Part model, mm, in its own coordinate system. A direction names the side the tool comes from. Coordinates: 2 decimals unless noted, no trailing zeros. Loops run counter-clockwise (first coordinate to the right, second up) from the corner with the lowest first, then second, coordinate; pieces in that order, holes last.
```python
from build123d import *

# Parameters (mm, degrees)
REVOLVE1_ANGLE      = 180
CUT_EXTRUDE1_DEPTH  = 173.874496063
BOSS_EXTRUDE1_DEPTH = 100
CUT_EXTRUDE2_DEPTH  = 161.866404199
CUT_REVOLVE2_ANGLE  = 90
SKETCH7_R           = 25
CUT_EXTRUDE3_DEPTH  = 161.866404199
SHELL1_T            = -2


with BuildPart() as part:
    # Sketch1 → Revolve1 (revolve)
    with BuildSketch(Plane(origin=(0, 0, 0), x_dir=(0, 0, -1), z_dir=(1, 0, 0))):
        with BuildLine():
            Line((0, -55), (0, 55))
            Line((0, 55), (-76.60153846, 55))
            ThreePointArc((-76.60153846, 55), (-94.301620847, 0), (-76.60153846, -55))
            Line((-76.60153846, -55), (0, -55))
        make_face()
    revolve(axis=Axis((0, -55, 0), (0, 1, 0)), revolution_arc=REVOLVE1_ANGLE)

    # Sketch2 → Cut-Extrude1 (cut, through all)
    with BuildSketch(Plane.XZ.offset(55)):
        Polygon((0, 0), (17.67766953, 17.67766953), (110.975280637, -75.619941577), (110.975280637, 155.951540754), (-110.127783366, 155.951540754), (-110.127783366, 0), align=None)
    extrude(amount=-CUT_EXTRUDE1_DEPTH, mode=Mode.SUBTRACT)

    # Sketch3 → Boss-Extrude1 (add)
    with BuildSketch(Plane(origin=(100, 0, 0), x_dir=(0, 0, -1), z_dir=(1, 0, 0))):
        Polygon((-71.226029464, -15), (-71.226029464, 15), (39.011689542, 30), (39.011689542, -30), align=None)
    extrude(amount=-BOSS_EXTRUDE1_DEPTH)

    # Sketch4 → Cut-Revolve1 (revolve, cut)
    with BuildSketch(Plane(origin=(0, 0, 0), x_dir=(0, 0, -1), z_dir=(1, 0, 0))):
        with BuildLine():
            Line((-59.361204271, 58.010752688), (-134.505556561, 58.010752688))
            ThreePointArc((-134.505556561, 58.010752688), (-146.4820541, 0), (-134.505556561, -58.010752688))
            Line((-134.505556561, -58.010752688), (-59.361204271, -58.010752688))
            ThreePointArc((-59.361204271, -58.010752688), (-83, 0), (-59.361204271, 58.010752688))
        make_face()
    revolve(axis=Axis((0, 0, 0), (0, 1, 0)), mode=Mode.SUBTRACT)

    # Sketch5 → Cut-Extrude2 (cut, through all)
    with BuildSketch(Plane.XZ.offset(55)):
        Polygon((0, 0), (70.470143291, 80), (-50.338034401, 80), (-50.338034401, 0), align=None)
    extrude(amount=-CUT_EXTRUDE2_DEPTH, mode=Mode.SUBTRACT)

    # Sketch6 → Cut-Revolve2 (revolve, cut)
    with BuildSketch(Plane(origin=(0, 0, 0), x_dir=(0, 0, -1), z_dir=(1, 0, 0))):
        with BuildLine():
            Line((-48.985500868, 65.760327742), (-101.43758046, 65.760327742))
            ThreePointArc((-101.43758046, 65.760327742), (-120.888392471, 0), (-101.43758046, -65.760327742))
            Line((-101.43758046, -65.760327742), (-48.985500868, -65.760327742))
            ThreePointArc((-48.985500868, -65.760327742), (-82, 0), (-48.985500868, 65.760327742))
        make_face()
    revolve(axis=Axis((0, 0, 0), (0, 1, 0)), revolution_arc=CUT_REVOLVE2_ANGLE, mode=Mode.SUBTRACT)

    # Sketch7 → Cut-Extrude3 (cut, through all)
    with BuildSketch(Plane.XZ.offset(55)):
        with Locations((0, -28)):
            Circle(SKETCH7_R)
    extrude(amount=-CUT_EXTRUDE3_DEPTH, mode=Mode.SUBTRACT)

    # Shell1
    shell1_openings = [part.faces().sort_by_distance(p)[0] for p in [
        (0, 0, -65.508602259),
        (25, 0, -28),
        (8.951286878, 39.236848999, 8.951286878),
        (8.951286878, -39.236848999, 8.951286878),
        (53.49764896, 22.71356766, 14.537622511),
        (53.49764896, -22.71356766, 14.537622511),
        (40.440192864, 39.71059478, -5.084853804),
        (40.440192864, -39.71059478, -5.084853804),
        (0, 0, -1.5),
        (25.1022253, 0, 28.496863072),
    ]]
    offset(amount=SHELL1_T, openings=shell1_openings, kind=Kind.INTERSECTION)


solid = part.part
```
Q1. Drop flat-ended pins along their axis: P1, Ø5, axis at y = 2.5, z = 9, coming from the +X side; P2, Ø4, axis at x = 78.5, y = -8.5, coming from the -Z side; P3, Ø12, axis at y = 42, z = 3.5, coming from the +X side; P4, Ø3, axis at x = 60, y = -2.5, coming from the +Z side. Give the stop position or say it passes through.
Q2. Tool access for faces 1 (the flat face through (82.6, 0.1, 0)), 2 (the cylindrical face through (24.994, 53.986, -28.55)), 3 (the flat face through (29, 53, -21)): list every direction of +Z, -Z, +X, -X, +Y, -Y with a clear straight run to the whole face (end or side of a thin tool).
Q3. Saw through at C-C (x = 73). List the corners of the cut face in (y, z), plus the area to 3 significant figures.
Q4. Saw through at A-A (z = -27). List the corners of the cut face in (x, y).
Q5. Saw through at B-B (x = 8). List the corners of the cut face in (y, z).
Q6. Probe line 1 (Y direction, x = 25.5, z = -8.5); line 2 (Z direction, x = 56, y = -8); line 3 (Z direction, x = 16, y = -31.5). List the from-to ranges inside material, lowest first.
Q7. Mould opens along Z. For faces 4 (the cylindrical face through (24.994, -54.014, -28.55)), 5 (the flat face through (80.2, 0.1, -2)), 6 (the flat face through (75.738, 22.894, 13.211)), 7 (the flat face through (0, 8, -81)) say: released by +Z, released by -Z, zero draft, split by the parting line, or undercut.
Q8. Saw through at D-D (x = 27). List the corners of the cut face in (y, z).
Checked values:
1. P1: stops at x = 81.71
1. P2: stops at z = -31.09
1. P3: passes through
1. P4: stops at z = 57.41
2. face 1: +Z, +X
2. face 2: -X, +Y, -Y
2. face 3: +Z, -X
3. outline: (-28.42, -27.42) arc R39.5 ccw to (28.42, -27.42) - (27.64, -21.64) arc R35.1 cw to (-27.64, -21.64) - close; (-21.31, 24.84) arc R32.73 cw to (21.31, 24.84) - (20.44, 31.26) arc R37.35 ccw to (-20.44, 31.26) - close
3. area: 486 mm2
4. outline: (24.98, -55) - (55.99, -55) arc R78.49 ccw to (62.36, -47.66) - (62.36, -44.09) arc R76.37 cw to (54.98, -53) - (24.98, -53) - close; (24.98, 53) - (54.98, 53) arc R76.37 cw to (62.36, 44.09) - (62.36, 47.66) arc R78.49 ccw to (55.99, 55) - (24.98, 55) - close; (70.9, -28.37) - (73.18, -28.37) arc R78.49 ccw to (73.18, 28.37) - (70.9, 28.37) arc R76.37 cw to start
5. outline: (-55, -61.64) arc R82.61 ccw to (55, -61.64) - (55, -51.69) - (53, -51.69) - (53, -60.73) arc R80.6 cw to (-53, -60.73) - (-53, -51.69) - (-55, -51.69) - close; (-55, -4.31) - (-53, -4.31) - (-53, 8) - (-55, 8) - close; (53, -4.31) - (55, -4.31) - (55, 8) - (53, 8) - close
6. line 1: y = -55 to -53, 53 to 55
6. line 2: z = -60.74 to -57.97, 56.57 to 59.36
6. line 3: z = -75.1 to -72.89
7. face 4: undercut
7. face 5: undercut
7. face 6: released by +Z
7. face 7: zero draft
8. outline: (-55, -55.99) arc R78.49 ccw to (55, -55.99) - (55, 8.36) - (53, 8.36) - (53, -54.98) arc R76.37 cw to (-53, -54.98) - (-53, 8.36) - (-55, 8.36) - close
